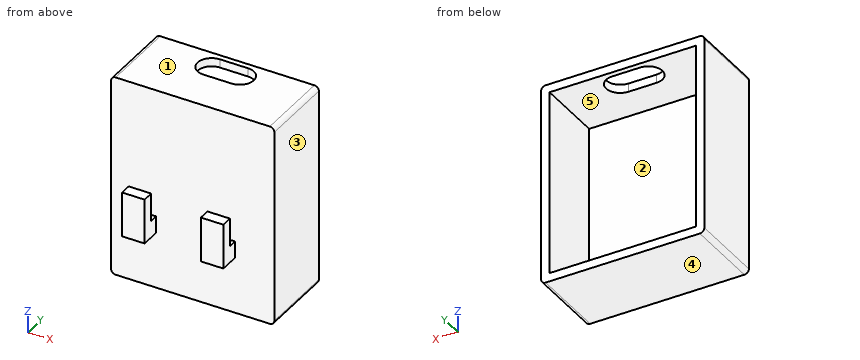
```python
from build123d import *

# Parameters (mm, degrees)
SKETCH1_W           = 29
SKETCH1_H           = 13.5
BOSS_EXTRUDE1_DEPTH = 36
SKETCH2_W           = 26
SKETCH2_H           = 33
CUT_EXTRUDE1_DEPTH  = 12
CUT_EXTRUDE2_DEPTH  = 1.5
FILLET1_R           = 0.8
SKETCH5_W           = 4
SKETCH5_H           = 8
BOSS_EXTRUDE2_DEPTH = 3.5
CUT_EXTRUDE3_REACH  = 49.011
SKETCH6_W           = 5
SKETCH6_H           = 1.5


with BuildPart() as part:
    # Sketch1 → Boss-Extrude1 (new body)
    with BuildSketch(Plane.XY):
        with Locations((14.5, -6.75)):
            Rectangle(SKETCH1_W, SKETCH1_H)
    extrude(amount=BOSS_EXTRUDE1_DEPTH)

    # Sketch2 → Cut-Extrude1 (cut)
    with BuildSketch(Plane(origin=(0, 0, 0), x_dir=(1, 0, 0), z_dir=(0, 1, 0))):
        with Locations((14.5, -18)):
            Rectangle(SKETCH2_W, SKETCH2_H)
    extrude(amount=-CUT_EXTRUDE1_DEPTH, mode=Mode.SUBTRACT)

    # Sketch3 → Cut-Extrude2 (cut)
    with BuildSketch(Plane.XY.offset(36)):
        with BuildLine():
            Line((12, -1), (17, -1))
            ThreePointArc((17, -1), (19.5, -3.5), (17, -6))
            Line((17, -6), (12, -6))
            ThreePointArc((12, -6), (9.5, -3.5), (12, -1))
        make_face()
    extrude(amount=-CUT_EXTRUDE2_DEPTH, mode=Mode.SUBTRACT)

    # Fillet1
    fillet1_edges = [part.edges().sort_by_distance(p)[0] for p in [
        (29, -6.75, 36),
        (0, -6.75, 36),
        (29, -6.75, 0),
        (0, -6.75, 0),
    ]]
    fillet(fillet1_edges, radius=FILLET1_R)

    # Sketch5 → Boss-Extrude2 (add)
    with BuildSketch(Plane.XZ.offset(13.5)):
        with Locations((20, 14)):
            Rectangle(SKETCH5_W, SKETCH5_H)
        with Locations((6, 14)):
            Rectangle(SKETCH5_W, SKETCH5_H)
    extrude(amount=BOSS_EXTRUDE2_DEPTH)

    # Cut-Extrude3: up to this face of the body (flat: up to its plane)
    cut_extrude3_end = Plane(part.part.faces().sort_by_distance((22, -15.25, 14))[0])
    # Sketch6 → Cut-Extrude3 (cut, up to the picked face)
    with BuildSketch(Plane.ZY.offset(-4), mode=Mode.PRIVATE) as cut_extrude3_sk1:
        with Locations((15.5, -14.25)):
            Rectangle(SKETCH6_W, SKETCH6_H)
    cut_extrude3_tool1 = split(extrude(cut_extrude3_sk1.sketch, amount=-CUT_EXTRUDE3_REACH, mode=Mode.PRIVATE), bisect_by=cut_extrude3_end, keep=Keep.BOTH, mode=Mode.PRIVATE)
    add(cut_extrude3_tool1.solids().sort_by(Axis((4, -14.25, 15.5), (1, 0, 0)))[0], mode=Mode.SUBTRACT)


solid = part.part
```
Part model, mm, in its own coordinate system. Face numbers are marked on the shaded views. A direction names the side the tool comes from. Give positions to 0.01 mm unless a question says otherwise; leave off trailing zeros. Order: outer loops, then holes, each group sorted by start corner. A loop starts at its lowest first (then second) coordinate and runs counter-clockwise, first axis right, second up. Notation, with made-up numbers: M 40,88 L 96,88 A23 ccw 96,115 Z; hole C 33.25,61.5 d10. An arc over 180 degrees is marked long. Use a Markdown table: item, result. Add a question column.
(1) Saw through at C-C, the plane y = -11.25. Give the cut face in (x, z).
(2) Mould opens along Z. For the marked faces 3, 4 and 5 say: +Z half, -Z half, draft (parallel to the pull), parting line (faces both ways), or undercut.
(3) Probe line 1 along Z through (x, y) = (10.25, -1); line 2 along X through (y, z) = (-1.25, 3.5); line 3 along Y through (x, z) = (20.5, 13.5). List the from-to ranges inside material, lowest first. Write a range as [from, to].
(4) 3-axis set-ups, long thin cutter, end or side, ignore diameter. For the marked faces 1 and 2: which of +Z, -Z, +X, -X, +Y, -Y reach the whole face in a straight line?
(5) Drop flat-ended pins along their axis: P1, Ø1.2, axis at x = 6.5, z = 16, coming from the +Y side; P2, Ø3, axis at y = -15.5, z = 13.5, coming from the -X side; P3, Ø0.6, axis at x = 20, y = -15.5, coming from the +Z side; P4, Ø14.5, axis at x = 11.5, z = 22, coming from the -Y side. Give the stop position or say it passes through.
(6) Saw through at B-B, the plane x = 18.5. Give the cut face in (y, z), and give its area (4 significant figures).
(7) Saw through at D-D, the plane z = 8. Give the cut face in (x, y).
(8) Saw through at A-A, the plane y = -3.5. Give the cut face in (x, z), and give its area (3 significant figures).
Answer key:
| question | item | result |
|---|---|---|
| 1 | outline | M 0,0.8 A0.8 ccw 0.8,0 L 28.2,0 A0.8 ccw 29,0.8 L 29,35.2 A0.8 ccw 28.2,36 L 0.8,36 A0.8 ccw 0,35.2 Z; hole M 1.5,1.5 L 27.5,1.5 L 27.5,34.5 L 1.5,34.5 Z |
| 2 | face 3 | draft |
| 2 | face 4 | -Z half |
| 2 | face 5 | undercut |
| 3 | line 1 | [0, 1.5], [34.5, 36] |
| 3 | line 2 | [0, 1.5], [27.5, 29] |
| 3 | line 3 | [-17, -15], [-13.5, -12] |
| 4 | face 1 | +Z, +X, -X, +Y, -Y |
| 4 | face 2 | +Y |
| 5 | P1 | y = -12 |
| 5 | P2 | x = 4 |
| 5 | P3 | z = 18 |
| 5 | P4 | y = -17 |
| 6 | outline | M -17,10 L -13.5,10 L -13.5,0 L 0,0 L 0,1.5 L -12,1.5 L -12,34.5 L -5.5,34.5 L -5.5,36 L -13.5,36 L -13.5,13 L -15,13 L -15,18 L -17,18 Z; M -1.5,34.5 L 0,34.5 L 0,36 L -1.5,36 Z |
| 6 | area | 104.5 mm^2 |
| 7 | outline | M 0,-13.5 L 29,-13.5 L 29,0 L 27.5,0 L 27.5,-12 L 1.5,-12 L 1.5,0 L 0,0 Z |
| 8 | outline | M 0,0.8 A0.8 ccw 0.8,0 L 28.2,0 A0.8 ccw 29,0.8 L 29,35.2 A0.8 ccw 28.2,36 L 19.5,36 L 19.5,34.5 L 27.5,34.5 L 27.5,1.5 L 1.5,1.5 L 1.5,34.5 L 9.5,34.5 L 9.5,36 L 0.8,36 A0.8 ccw 0,35.2 Z |
| 8 | area | 170 mm^2 |
